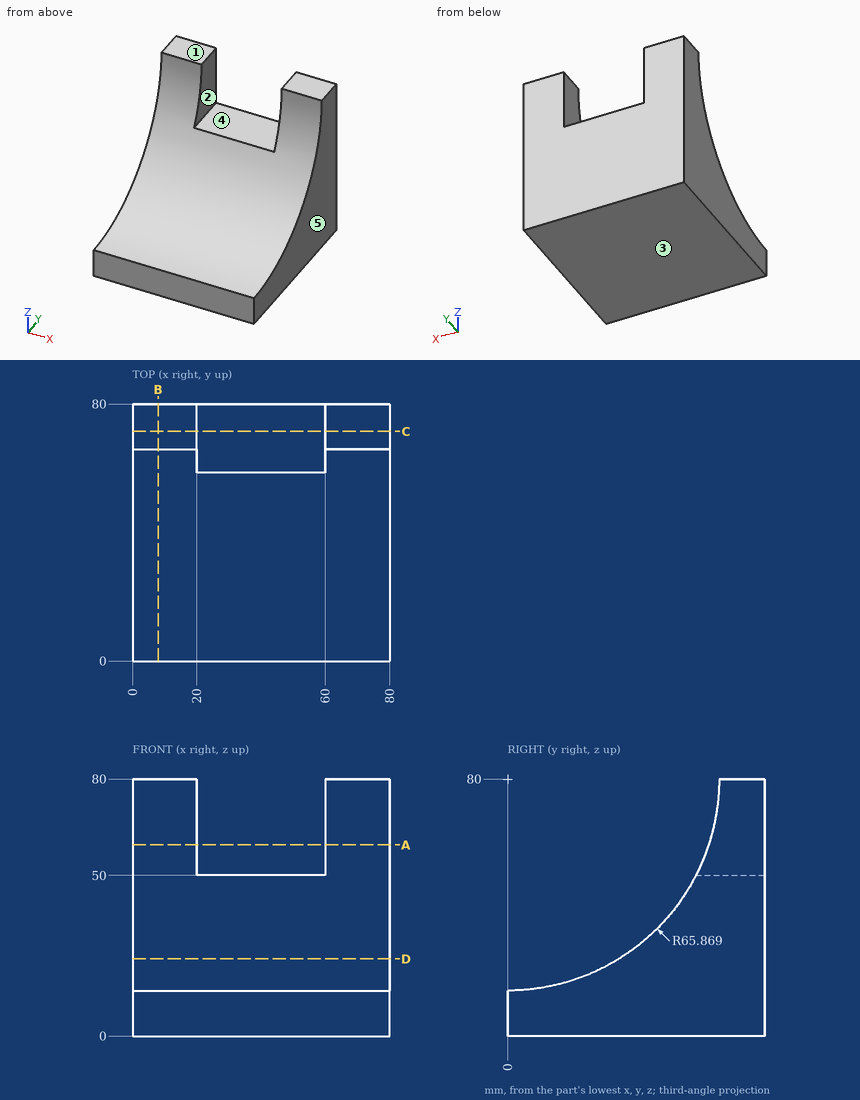
Could you check a few things on this drawing? It's one solid part, dimensions in mm from its lowest x, y, z. A direction names the side the tool comes from. Round coordinates to 2 decimals unless told otherwise and drop trailing zeros. Order: outer loops, then holes, each group sorted by start corner. A loop starts at its lowest first (then second) coordinate and runs counter-clockwise, first axis right, second up. Notation, with made-up numbers: M -19,49 L -5,49 A36 cw -5,84 Z; hole C 66.5,36.25 d8. An arc over 180 degrees is marked long. One line per item, written item: value.
(1) Imagine slicing it at A-A (z = 59.5). Write out the boundary of the cut face in (x, y).
Ans:
outline: M 0,62.6 L 20,62.6 L 20,80 L 0,80 Z; M 60,62.6 L 80,62.6 L 80,80 L 60,80 Z
(2) I need wall thicknesses on line 1 along X through (y, z) = (77, 66); line 2 along Z through (x, y) = (32.5, 67.5); line 3 along Y through (x, z) = (71, 21). Which ranges of each line are inside material? Lowest first, please. Write a range as from..to.
Ans:
line 1: x = 0..20, 60..80
line 2: z = 0..50
line 3: y = 29.29..80
(3) Imagine slicing it at C-C (y = 71.5). Write out the boundary of the cut face in (x, z), and give its area (3 significant figures).
Ans:
outline: M 0,0 L 80,0 L 80,80 L 60,80 L 60,50 L 20,50 L 20,80 L 0,80 Z
area: 5,200 mm^2
(4) If we mould it in two halves opening along X, with no side actions, what happens to the marked faces 3, 4 and 5? For each: released by +X, released by -X, zero draft, split by the parting line, or undercut.
Ans:
face 3: zero draft
face 4: undercut
face 5: released by +X
(5) Imagine slicing it at D-D (z = 24). Write out the boundary of the cut face in (x, y).
Ans:
outline: M 0,34.68 L 80,34.68 L 80,80 L 0,80 Z
(6) Which directions (+Z, -Z, +X, -X, +Y, -Y) give clear straight access to the entire face, cutting with the end or side of a thin tool? Please do the marked faces 1 and 2.
Ans:
face 1: +Z, +X, -X, +Y, -Y
face 2: +Z, +Y, -Y
(7) Imagine slicing it at B-B (x = 8). Write out the boundary of the cut face in (y, z), and give its area (3 significant figures).
Ans:
outline: M 0,0 L 80,0 L 80,80 L 65.87,80 A65.87 cw 0,14.13 Z
area: 2,990 mm^2
(8) I'm going to push flat-ended pins straight in: P1, Ø23.5, axis at y = 71.5, z = 69, coming from the -X side; P2, Ø17, axis at x = 36.5, y = 70.5, coming from the +Z side. Where does each tip first touch, or does it pass through?
Ans:
P1: stops at x = 0
P2: stops at z = 50
